```python
from build123d import *

# Parameters (mm, degrees)
SKETCH1_W           = 152.4
SKETCH1_H           = 101.6
BOSS_EXTRUDE1_DEPTH = 152.4
CUT_EXTRUDE2_DEPTH  = 152.4
SKETCH7_W           = 139.7
SKETCH7_H           = 127
CUT_EXTRUDE3_DEPTH  = 88.9
SKETCH8_R           = 3.175
CUT_EXTRUDE4_DEPTH  = 12.7
SKETCH9_R           = 3.175
CUT_EXTRUDE5_DEPTH  = 12.7


with BuildPart() as part:
    # Sketch1 → Boss-Extrude1 (new body)
    with BuildSketch(Plane.XY):
        with Locations((76.2, 50.8)):
            Rectangle(SKETCH1_W, SKETCH1_H)
    extrude(amount=BOSS_EXTRUDE1_DEPTH)

    # Sketch6 → Cut-Extrude2 (cut)
    with BuildSketch(Plane.XY.offset(152.4)):
        Polygon((104.436678767, 101.6), (38.1, 101.6), (152.4, 38.1), (152.4, 101.6), (104.590197544, 101.6), align=None)
    extrude(amount=-CUT_EXTRUDE2_DEPTH, mode=Mode.SUBTRACT)

    # Sketch7 → Cut-Extrude3 (cut)
    with BuildSketch(Plane(origin=(0, 101.6, 0), x_dir=(1, 0, 0), z_dir=(0, 1, 0))):
        with Locations((76.2, -76.2)):
            Rectangle(SKETCH7_W, SKETCH7_H)
    extrude(amount=-CUT_EXTRUDE3_DEPTH, mode=Mode.SUBTRACT)

    # Sketch8 → Cut-Extrude4 (cut)
    with BuildSketch(Plane(origin=(0, 101.6, 0), x_dir=(1, 0, 0), z_dir=(0, 1, 0))):
        with Locations((12.7, -146.05)):
            Circle(SKETCH8_R)
        with Locations((12.7, -6.35)):
            Circle(SKETCH8_R)
    extrude(amount=-CUT_EXTRUDE4_DEPTH, mode=Mode.SUBTRACT)

    # Sketch9 → Cut-Extrude5 (cut)
    with BuildSketch(Plane(origin=(52.117924528, 93.812264151, 0), x_dir=(0.874157276, -0.485642931, 0), z_dir=(0.485642931, 0.874157276, 0))):
        with Locations((102.018573203, -146.05)):
            Circle(SKETCH9_R)
        with Locations((102.018573203, -6.604)):
            Circle(SKETCH9_R)
    extrude(amount=-CUT_EXTRUDE5_DEPTH, mode=Mode.SUBTRACT)


solid = part.part
```
Read the model definition and answer for the solid it produces. Units are mm, in the model's axes. A direction names the side the tool comes from. Give positions to 0.01 mm unless a question says otherwise; leave off trailing zeros. Order: outer loops, then holes, each group sorted by start corner. A loop starts at its lowest first (then second) coordinate and runs counter-clockwise, first axis right, second up. Notation, with made-up numbers: (41.5, 31) -> (53.5, 31) arc R27 cw to (53.5, 65) -> close; hole circle Ø8 at (-37, 33). An arc over 180 degrees is marked (long way). Write item = value, one per line.
1. A cutting plane is placed at A-A, the plane x = 12.7. Write down the section's boundary in (y, z) (3 decimals).
Numbers:
outline = (0, 0) -> (101.6, 0) -> (101.6, 3.175) -> (88.9, 3.175) -> (88.9, 9.525) -> (101.6, 9.525) -> (101.6, 12.7) -> (12.7, 12.7) -> (12.7, 139.7) -> (101.6, 139.7) -> (101.6, 142.875) -> (88.9, 142.875) -> (88.9, 149.225) -> (101.6, 149.225) -> (101.6, 152.4) -> (0, 152.4) -> close
2. A cutting plane is placed at B-B, the plane y = 24. Write down the section's boundary in (x, z).
Numbers:
outline = (0, 0) -> (152.4, 0) -> (152.4, 152.4) -> (0, 152.4) -> close; hole (6.35, 12.7) -> (146.05, 12.7) -> (146.05, 139.7) -> (6.35, 139.7) -> close
3. A cutting plane is placed at D-D, the plane z = 52. Write down the section's boundary in (x, y), and give its area (3 significant figures).
Numbers:
outline = (0, 0) -> (152.4, 0) -> (152.4, 38.1) -> (146.05, 41.63) -> (146.05, 12.7) -> (6.35, 12.7) -> (6.35, 101.6) -> (0, 101.6) -> close
area = 2,670 mm²
4. Given pin 1 (5 mm diameter, centred on x = 89, z = 133.5, fed in from -Y); pin 2 (4 mm diameter, centred on x = 12.7, z = 6.35, fed in from +Y); pin 3 (10 mm diameter, centred on y = 85, z = 120.5, fed in from +X); pin 4 (12 mm diameter, centred on x = 123.5, y = 64, fed in from -Z) (3 decimals), each flat-ended and moving along its own axis, determine where each tip first touches the part or whether it passes through.
Numbers:
pin_1 = 0
pin_2 = 88.9
pin_3 = 6.35
pin_4 = through
5. The mould has two halves that part along Z. Classify faces 4 (the face through (58, 40, 0)), 5 (the face through (135.09, 33.19, 6.56)), 6 (the face through (58, 40, 152.4)): +Z half, -Z half, draft (parallel to the pull), parting line (faces both ways), or undercut.
Numbers:
face_4 = -Z half
face_5 = undercut
face_6 = +Z half
6. A cutting plane is placed at C-C, the plane y = 52.5. Write down the section's boundary in (x, z), and give its area (3 significant figures).
Numbers:
outline = (0, 0) -> (126.48, 0) -> (126.48, 12.7) -> (6.35, 12.7) -> (6.35, 139.7) -> (126.48, 139.7) -> (126.48, 152.4) -> (0, 152.4) -> close
area = 4,020 mm²
7. For faces 1 (the face through (135.09, 33.19, 146.01)), 2 (the face through (0, 50, 75)), 3 (the face through (60, 48, 12.7)), determine the directions among +Z, -Z, +X, -X, +Y, -Y from which every point of the face is accessible in a straight line to the end or side of a thin tool.
Numbers:
face_1 = none
face_2 = +Z, -Z, -X, +Y, -Y
face_3 = +Y
8. Straight lines are drawn through the part: line 1 along Z through (x, y) = (12.7, 97.5) (3 decimals); line 2 along Z through (x, y) = (86, 33.5); line 3 along Z through (x, y) = (12, 98). For each, find the intervals that lie inside material, in ascending order.
Numbers:
line_1 = 0 to 3.175, 9.525 to 12.7, 139.7 to 142.875, 149.225 to 152.4
line_2 = 0 to 12.7, 139.7 to 152.4
line_3 = 0 to 3.25, 9.45 to 12.7, 139.7 to 142.95, 149.15 to 152.4
